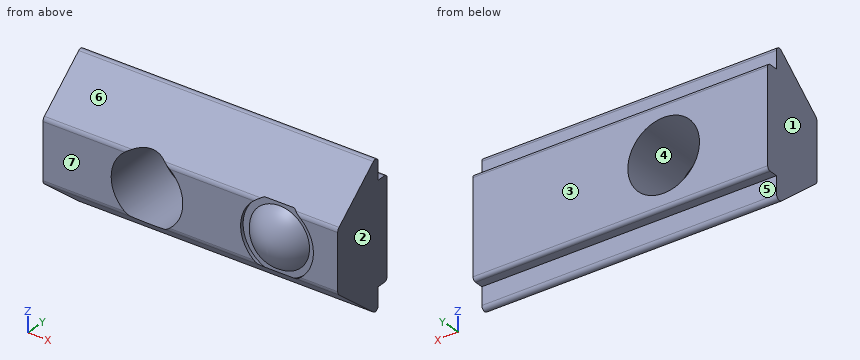
```python
from build123d import *

# Parameters (mm, degrees)
BOSS_EXTRUDE1_DEPTH = 17
FILLET1_R           = 0.3
FILLET2_R           = 0.2
SKETCH2_W           = 2.1
SKETCH2_H           = 0.2
TAPPED_HOLE1_D      = 4.134


with BuildPart() as part:
    # Sketch1 → Boss-Extrude1 (new body)
    with BuildSketch(Plane(origin=(-6, 0, 0), x_dir=(0, 0, -1), z_dir=(1, 0, 0))):
        with BuildLine():
            Line((2.9, 0), (-2.9, 0))
            Line((-2.9, 0), (-2.9, -0.7))
            Line((-2.9, -0.7), (-3.92, -0.7))
            ThreePointArc((-3.92, -0.7), (-4.128228295, -0.832322075), (-4.096863547, -1.077034982))
            Line((-4.096863547, -1.077034982), (-1.75, -3.9))
            Line((-1.75, -3.9), (1.75, -3.9))
            Line((1.75, -3.9), (4.096863547, -1.077034982))
            ThreePointArc((4.096863547, -1.077034982), (4.128228295, -0.832322075), (3.92, -0.7))
            Line((3.92, -0.7), (2.9, -0.7))
            Line((2.9, -0.7), (2.9, 0))
        make_face()
    extrude(amount=BOSS_EXTRUDE1_DEPTH)

    # Fillet1
    fillet1_edges = [part.edges().sort_by_distance(p)[0] for p in [
        (2.5, -3.9, -1.75),
        (2.5, -3.9, 1.75),
    ]]
    fillet(fillet1_edges, radius=FILLET1_R)

    # Fillet2
    fillet2_edges = [part.edges().sort_by_distance(p)[0] for p in [
        (2.5, 0, 2.9),
        (2.5, 0, -2.9),
    ]]
    fillet(fillet2_edges, radius=FILLET2_R)

    # Sketch2 → Cut-Revolve1 (revolve, cut)
    with BuildSketch(Plane(origin=(7.5, 0, 0), x_dir=(0, 0, -1), z_dir=(1, 0, 0))):
        with Locations((1.05, -3.8)):
            Rectangle(SKETCH2_W, SKETCH2_H)
    revolve(axis=Axis((7.5, 1.665548573, 0), (0, -1, 0)), mode=Mode.SUBTRACT)

    # Sketch3 → Revolve1 (revolve)
    with BuildSketch(Plane(origin=(7.5, 0, 0), x_dir=(0, 0, -1), z_dir=(1, 0, 0))):
        with BuildLine():
            Line((1.732050808, -3.7), (0, -3.7))
            Line((0, -3.7), (0, -4.7))
            ThreePointArc((0, -4.7), (1, -4.432050808), (1.732050808, -3.7))
        make_face()
    revolve(axis=Axis((7.5, 0, 0), (0, -1, 0)))

    # Tapped Hole1 (through all)
    with Locations(Plane(origin=(0, 0, 0), x_dir=(1, 0, 0), z_dir=(0, 1, 0))):
        with Locations((0, 0)):
            Hole(TAPPED_HOLE1_D / 2)


solid = part.part
```
Input: part model. Units: mm. Frame: model coordinates. Face numbers are marked on the shaded views. A direction names the side the tool comes from. Coordinates: 2 decimals unless noted, no trailing zeros. Loops run counter-clockwise (first coordinate to the right, second up) from the corner with the lowest first, then second, coordinate; pieces in that order, holes last.
Q1. Set-up query: the marked faces 5, 6 and 7. Return all of +Z, -Z, +X, -X, +Y, -Y with unobstructed straight access to the full face (end or side cutting, diameter ignored); none if empty.
Results are:
face 5: -Z, +X, -X, +Y
face 6: +Z, +X, -X, -Y
face 7: +Z, -Z, -X, -Y
Q2. Mould query, pull axis X, two halves, no side actions, for the marked faces 1, 2, 3 and 4. Classes: +X half, -X half, draft (parallel to the pull), parting line (faces both ways), or undercut.
Results are:
face 1: -X half
face 2: +X half
face 3: draft
face 4: undercut
Q3. Line query: line 1 along Y through (x, z) = (-2.75, 0.25); line 2 along X through (y, z) = (-3.05, -1.5); line 3 along Z through (x, y) = (0, -2.8). Output: solid intervals per line, ascending.
Results are:
line 1: y = -3.9 to 0
line 2: x = -6 to -1.42, 1.42 to 11
line 3: z = -2.66 to -2.07, 2.07 to 2.66
Q4. Section A-A, the plane z = 0. Return the cut outline in (x, y), and give its area (3 significant figures).
Results are:
outline: (-6, -3.9) - (-2.07, -3.9) - (-2.07, 0) - (-6, 0) - close; (2.07, -3.9) - (5.4, -3.9) - (5.4, -3.7) - (5.77, -3.7) arc R2 ccw to (9.23, -3.7) - (9.6, -3.7) - (9.6, -3.9) - (11, -3.9) - (11, 0) - (2.07, 0) - close
area: 51.8 mm2
Q5. Section B-B, the plane x = -4. Return the cut outline in (y, z), and give its area (3 significant figures).
Results are:
outline: (-3.9, -1.61) arc R0.3 ccw to (-3.79, -1.84) - (-1.08, -4.1) arc R0.23 ccw to (-0.7, -3.92) - (-0.7, -2.9) - (-0.2, -2.9) arc R0.2 ccw to (0, -2.7) - (0, 2.7) arc R0.2 ccw to (-0.2, 2.9) - (-0.7, 2.9) - (-0.7, 3.92) arc R0.23 ccw to (-1.08, 4.1) - (-3.79, 1.84) arc R0.3 ccw to (-3.9, 1.61) - close
area: 23.6 mm2
Q6. Contact query for flat-ended pins moving along their axis: pin 1 (3.5 mm diameter, centred on x = 0, z = 0, fed in from +Y); pin 2 (1.1 mm diameter, centred on x = 10, z = 0, fed in from -Y); pin 3 (3.5 mm diameter, centred on x = 4.5, z = 0.5, fed in from -Y); pin 4 (0.8 mm diameter, centred on x = 1.5, z = -3.5, fed in from +Y). Output: stop coordinate, or through.
Results are:
pin 1: passes through
pin 2: stops at y = -3.9
pin 3: stops at y = -4.23
pin 4: stops at y = -0.7
Q7. Section C-C, the plane x = 0. Return the cut outline in (y, z).
Results are:
outline: (-3.52, -2.07) - (-1.08, -4.1) arc R0.23 ccw to (-0.7, -3.92) - (-0.7, -2.9) - (-0.2, -2.9) arc R0.2 ccw to (0, -2.7) - (0, -2.07) - close; (-3.52, 2.07) - (0, 2.07) - (0, 2.7) arc R0.2 ccw to (-0.2, 2.9) - (-0.7, 2.9) - (-0.7, 3.92) arc R0.23 ccw to (-1.08, 4.1) - close
Q8. Section D-D, the plane y = -1.4. Return the cut outline in (x, z).
Results are:
outline: (-6, -3.83) - (11, -3.83) - (11, 3.83) - (-6, 3.83) - close; hole circle Ø4.13 at (0, 0)
